from build123d import *

# Parameters (mm, degrees)
PAD_DEPTH         = 149.225
PAD001_DEPTH      = 3.175
PAD002_DEPTH      = 3.175
POCKET_DEPTH      = 155.6014
POCKET_DEPTH_BACK = 22.226
SKETCH004_W       = 19.05
SKETCH004_H       = 9.525
SKETCH004_H_2     = 6.35
POCKET001_DEPTH   = 3.175
SKETCH005_W       = 41.275
SKETCH005_H       = 19.05
POCKET002_DEPTH   = 111.126


with BuildPart() as part:
    # Sketch → Pad (new body)
    with BuildSketch(Plane.XY):
        Polygon((-133.3754, 0), (-133.3754, 91.9226), (-114.173, 111.125), (0, 111.125), (0, 0), (-3.175, 0), (-3.175, 107.95), (-112.857872, 107.95), (-130.2004, 90.607472), (-130.2004, 0), align=None)
    extrude(amount=PAD_DEPTH)

    # Sketch001 (on Face12 of Pad) → Pad001 (join)
    with BuildSketch(Plane.XY.offset(149.225)):
        Polygon((-114.173, 111.125), (0, 111.125), (0, 0), (-133.3754, 0), (-133.3754, 91.9226), align=None)
    extrude(amount=PAD001_DEPTH)

    # Sketch002 (on Face4 of Pad001) → Pad002 (join)
    with BuildSketch(Plane(origin=(0, 0, 0), x_dir=(1, 0, 0), z_dir=(0, 0, -1))):
        with BuildLine():
            Line((-130.2004, 0), (-130.2004, -90.607472))
            Line((-130.2004, -90.607472), (-112.857872, -107.95))
            Line((-112.857872, -107.95), (-3.175, -107.95))
            Line((-3.175, -107.95), (-3.175, 0))
            Line((-3.175, 0), (6.0325, 0))
            Line((6.0325, 0), (6.0325, -5.08))
            ThreePointArc((6.0325, -5.08), (6.53345, -7.279705), (7.9375, -9.045574))
            Line((7.9375, -9.045574), (7.9375, -33.782))
            ThreePointArc((7.9375, -33.782), (11.1125, -36.957), (14.2875, -33.782))
            Line((14.2875, -33.782), (14.2875, -9.045574))
            ThreePointArc((14.2875, -9.045574), (15.69155, -7.279705), (16.1925, -5.08))
            Line((16.1925, -5.08), (16.1925, 0))
            Line((16.1925, 0), (22.225, 0))
            Line((22.225, 0), (22.225, -101.4984))
            ThreePointArc((-3.175, -126.8984), (14.785512, -119.458912), (22.225, -101.4984))
            Line((-130.2004, -126.8984), (-3.175, -126.8984))
            ThreePointArc((-155.6004, -101.4984), (-148.160912, -119.458912), (-130.2004, -126.8984))
            Line((-155.6004, 0), (-155.6004, -101.4984))
            Line((-155.6004, 0), (-147.9804, 0))
            Line((-147.9804, -5.08), (-147.9804, 0))
            ThreePointArc((-147.9804, -5.08), (-147.47945, -7.279705), (-146.0754, -9.045574))
            Line((-146.0754, -9.045574), (-146.0754, -33.782))
            ThreePointArc((-146.0754, -33.782), (-142.9004, -36.957), (-139.7254, -33.782))
            Line((-139.7254, -33.782), (-139.7254, -9.045574))
            ThreePointArc((-139.7254, -9.045574), (-138.32135, -7.279705), (-137.8204, -5.08))
            Line((-137.8204, -5.08), (-137.8204, 0))
            Line((-137.8204, 0), (-130.2004, 0))
        make_face()
        with BuildLine():
            ThreePointArc((14.2875, -59.845574), (11.1125, -50.8), (7.9375, -59.845574))
            Line((7.9375, -59.845574), (7.9375, -84.582))
            ThreePointArc((7.9375, -84.582), (11.1125, -87.757), (14.2875, -84.582))
            Line((14.2875, -84.582), (14.2875, -59.845574))
        make_face(mode=Mode.SUBTRACT)
        with BuildLine():
            ThreePointArc((-139.7254, -59.845574), (-142.9004, -50.8), (-146.0754, -59.845574))
            Line((-146.0754, -59.845574), (-146.0754, -84.582))
            ThreePointArc((-146.0754, -84.582), (-142.9004, -87.757), (-139.7254, -84.582))
            Line((-139.7254, -84.582), (-139.7254, -59.845574))
        make_face(mode=Mode.SUBTRACT)
    extrude(amount=-PAD002_DEPTH)

    # Sketch003 (on Face48 of Pad002) → Pocket (cut, two sides)
    with BuildSketch(Plane.YZ) as pocket_sk:
        with BuildLine():
            ThreePointArc((25.200781, 3.175), (17.960512, 17.960512), (3.175, 25.200781))
            ThreePointArc((0, 28.375781), (0.929936, 26.130717), (3.175, 25.200781))
            Line((0, 28.375781), (-5, 28.375781))
            Line((-5, 28.375781), (-5, -5))
            Line((-5, -5), (28.375781, -5))
            Line((28.375781, -5), (28.375781, 0))
            ThreePointArc((25.200781, 3.175), (26.130717, 0.929936), (28.375781, 0))
        make_face()
    extrude(amount=-POCKET_DEPTH, mode=Mode.SUBTRACT)
    extrude(pocket_sk.sketch, amount=POCKET_DEPTH_BACK, mode=Mode.SUBTRACT)

    # Sketch004 (on Face38 of Pocket) → Pocket001 (cut)
    with BuildSketch(Plane.YZ):
        with Locations((37.592, 93.6625)):
            Rectangle(SKETCH004_W, SKETCH004_H)
        with Locations((82.042, 92.075)):
            Rectangle(SKETCH004_W, SKETCH004_H_2)
    extrude(amount=-POCKET001_DEPTH, mode=Mode.SUBTRACT)

    # Sketch005 (on Face39 of Pocket001) → Pocket002 (cut, through all)
    with BuildSketch(Plane(origin=(0, 111.125, 0), x_dir=(-1, 0, 0), z_dir=(0, 1, 0))):
        with Locations((82.5627, 128.6002)):
            Rectangle(SKETCH005_W, SKETCH005_H)
    extrude(amount=-POCKET002_DEPTH, mode=Mode.SUBTRACT)


solid = part.part
For this review, take the finished solid that the model builds, in its own axes (mm). A direction names the side the tool comes from. Round coordinates to 2 decimals unless told otherwise and drop trailing zeros. Order: outer loops, then holes, each group sorted by start corner. A loop starts at its lowest first (then second) coordinate and runs counter-clockwise, first axis right, second up. Notation, with made-up numbers: (-28.75, 31) -> (16.25, 31) arc R7 cw to (16.25, 39) -> close; hole circle Ø3 at (-22, 87). An arc over 180 degrees is marked (long way). Put each result on its own line as item: value.
Q1. Add section B-B on y = 55.88. Write out the cut boundary in (x, z) (1 decimal).
Check result:
outline: (-155.6, 0) -> (-148, 0) -> (-148, 3.2) -> (-155.6, 3.2) -> close; (-137.8, 0) -> (-130.2, 0) -> (-130.2, 149.2) -> (-3.2, 149.2) -> (-3.2, 0) -> (6, 0) -> (6, 3.2) -> (0, 3.2) -> (0, 152.4) -> (-133.4, 152.4) -> (-133.4, 3.2) -> (-137.8, 3.2) -> close; (16.2, 0) -> (22.2, 0) -> (22.2, 3.2) -> (16.2, 3.2) -> close
Q2. Add section D-D on z = 72.5. Write out the cut boundary in (x, y) (3 decimals), plus the area to 3 significant figures.
Check result:
outline: (-133.375, 0) -> (-130.2, 0) -> (-130.2, 90.607) -> (-112.858, 107.95) -> (-3.175, 107.95) -> (-3.175, 0) -> (0, 0) -> (0, 111.125) -> (-114.173, 111.125) -> (-133.375, 91.923) -> close
area: 1,070 mm2
Q3. Mouldability with a two-part tool opening along X and no side actions: class faces 4 (the flat face through (-121.41, 99.4, 73.57)), 5 (the flat face through (-66, 56, 152.4)), 6 (the flat face through (-133.375, 45, 77)), 7 (the cylindrical face through (11.288, 50.803, 1.565)) as pulls with the +X half, pulls with the -X half, needs draft (parallel to the pull), parting line crosses it, or undercut.
Check result:
face 4: undercut
face 5: needs draft
face 6: pulls with the -X half
face 7: undercut
Q4. Add section C-C on x = -65. Write out the cut boundary in (y, z) (3 decimals), plus the area to 3 significant figures.
Check result:
outline: (0, 149.225) -> (107.95, 149.225) -> (107.95, 138.125) -> (111.125, 138.125) -> (111.125, 152.4) -> (0, 152.4) -> close; (107.95, 0) -> (126.898, 0) -> (126.898, 3.175) -> (111.125, 3.175) -> (111.125, 119.075) -> (107.95, 119.075) -> close
area: 816 mm2
Q5. Insertion check: pin 1 Ø8 at (x, z) = (-32, 39.5) entering from -Y; pin 2 Ø2.5 at (y, z) = (110, 130) entering from +X; pin 3 Ø3.5 at (x, z) = (-1.5, 95) entering from +Y (3 decimals). Each pin has a flat end and moves straight along its axis. Give the tip position at first contact, or say it passes through.
Check result:
pin 1: y = 107.95
pin 2: x = 0
pin 3: y = 111.125
Q6. Add section A-A on y = 39.5. Write out the cut boundary in (x, z) (3 decimals).
Check result:
outline: (-155.6, 0) -> (-130.2, 0) -> (-130.2, 149.225) -> (-3.175, 149.225) -> (-3.175, 98.425) -> (0, 98.425) -> (0, 152.4) -> (-133.375, 152.4) -> (-133.375, 3.175) -> (-155.6, 3.175) -> close; (-3.175, 0) -> (22.225, 0) -> (22.225, 3.175) -> (0, 3.175) -> (0, 88.9) -> (-3.175, 88.9) -> close
Q7. For probe 1 along X at (y, z) = (55.88, 1.9) (1 decimal); probe 2 along X at (y, z) = (55, 1) (3 decimals); probe 3 along X at (y, z) = (13.5, 117) (3 decimals), list the stretches that pass through material, from the lowest coordinate up. Write a range as [from, to].
Check result:
probe 1: [-155.6, -148], [-137.8, -130.2], [-3.2, 6], [16.2, 22.2]
probe 2: [-155.6, -147.904], [-137.897, -130.2], [-3.175, 6.109], [16.116, 22.225]
probe 3: [-133.375, -130.2], [-3.175, 0]
Q8. Machinability: for faces 1 (the flat face through (-58, 111.125, 77)), 2 (the flat face through (-57, 107.95, 74)), 3 (the flat face through (0, 56, 77)), which of the approach directions +Z, -Z, +X, -X, +Y, -Y give a long, thin tool a straight path to every point of the face, cutting with its end or side? Answer none if there is none.
Check result:
face 1: +Z, +X, -X, +Y
face 2: -Z, -Y
face 3: +Z, +X, +Y, -Y
